from build123d import *

# Parameters (mm, degrees)
F0_R     = 51.347904
F1_DEPTH = 5.08
F2_R     = 9.265386
F3_DEPTH = 38.862
F4_R     = 3.740808
F5_DEPTH = 28.702


with BuildPart() as f1:
    # F0 (on Front) → F1 (new body)
    with BuildSketch(Plane.XZ):
        Circle(F0_R)
    extrude(amount=F1_DEPTH)

    # F2 (on Front) → F3 (join)
    with BuildSketch(Plane.XZ):
        Circle(F2_R)
    extrude(amount=F3_DEPTH)

    # F4 (on face) → F5 (cut)
    with BuildSketch(Plane.XZ.offset(38.862)):
        Circle(F4_R)
    extrude(amount=-F5_DEPTH, mode=Mode.SUBTRACT)


solid = f1.part
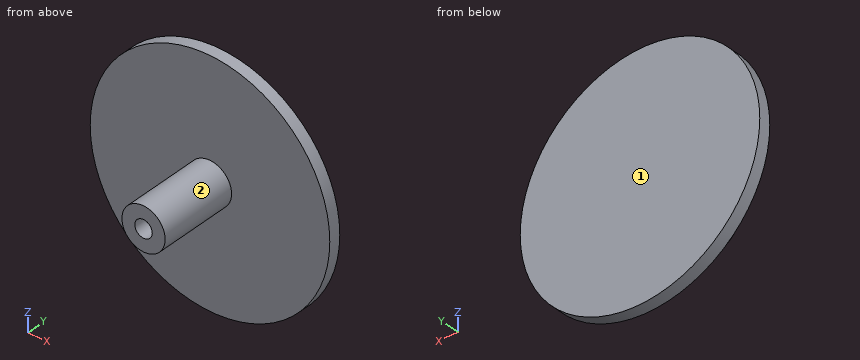
Source: CAD feature listing. Evaluate the final solid. Frame: model axes, mm. Face numbers are marked on the shaded views. A direction names the side the tool comes from. Give positions to 0.01 mm unless a question says otherwise; leave off trailing zeros. Write each loop counter-clockwise with the first axis right and the second up, starting at its lowest first coordinate (ties: lowest second). Pieces come first, ordered by that corner, then holes. Notation, with made-up numbers: M -13,9 L 24,9 A17 ccw 24,27 Z; hole C 81,22 d6. An arc over 180 degrees is marked long. Return JSON: item names as keys, results as strings. Group by question number.
1) Material intervals for line 1 along Z through (x, y) = (0, -28); line 2 along Y through (x, z) = (-17.5, -1); line 3 along Z through (x, y) = (41, -2.5), sorted ascending. Write a range as [from, to].
2) Set-up query: the marked faces 1 and 2. Return all of +Z, -Z, +X, -X, +Y, -Y with unobstructed straight access to the full face (end or side cutting, diameter ignored); none if empty.
3) Cut plane A-A, the plane z = 0. Output: boundary loops of the cut face in (x, y), plus the area to 3 significant figures.
4) Cut plane C-C, the plane y = -12.5. Output: boundary loops of the cut face in (x, z).
5) Cut plane D-D, the plane x = 32. Output: boundary loops of the cut face in (y, z), plus the area to 3 significant figures.
6) Cut plane B-B, the plane x = 0. Output: boundary loops of the cut face in (y, z), plus the area to 3 significant figures.
7) Pin query (flat end, axial travel): P1, Ø8, axis at y = -10.5, z = 19.5, coming from the -X side; P2, Ø12, axis at y = -6, z = 26, coming from the -X side; P3, Ø4, axis at x = -8.5, z = -37.5, coming from the -Y side; P4, Ø5, axis at x = 8, y = -18, coming from the +Z side. Return the tip coordinate at first contact, or that it passes through.
Recorded:
{
 "1": {"line 1": "z = [-9.27, -3.74], [3.74, 9.27]", "line 2": "y = [-5.08, 0]", "line 3": "z = [-30.91, 30.91]"},
 "2": {"face 1": "+Z, -Z, +X, -X, +Y", "face 2": "-Y"},
 "3": {"outline": "M -51.35,-5.08 L -9.27,-5.08 L -9.27,-38.86 L -3.74,-38.86 L -3.74,-10.16 L 3.74,-10.16 L 3.74,-38.86 L 9.27,-38.86 L 9.27,-5.08 L 51.35,-5.08 L 51.35,0 L -51.35,0 Z", "area": "933 mm²"},
 "4": {"outline": "C 0,0 d18.53; hole C 0,0 d7.48"},
 "5": {"outline": "M -5.08,-40.16 L 0,-40.16 L 0,40.16 L -5.08,40.16 Z", "area": "408 mm²"},
 "6": {"outline": "M -38.86,-9.27 L -5.08,-9.27 L -5.08,-51.35 L 0,-51.35 L 0,51.35 L -5.08,51.35 L -5.08,9.27 L -38.86,9.27 L -38.86,3.74 L -10.16,3.74 L -10.16,-3.74 L -38.86,-3.74 Z", "area": "933 mm²"},
 "7": {"P1": "passes through", "P2": "stops at x = -47.26", "P3": "stops at y = -5.08", "P4": "stops at z = 7.46"}
}
